Part model, mm, in its own coordinate system. A direction names the side the tool comes from. Give positions to 0.01 mm unless a question says otherwise; leave off trailing zeros. Write each loop counter-clockwise with the first axis right and the second up, starting at its lowest first coordinate (ties: lowest second). Pieces come first, ordered by that corner, then holes.
```python
from build123d import *

# Parameters (mm, degrees)
F0_W      = 38.862
F0_H      = 38.862
F1_DEPTH  = 10.668
F2_SIZE   = 7.62
F4_DEPTH  = 6.35
F5_SIZE   = 5.08
F7_DEPTH  = 6.35
F8_R      = 10.9982
F9_DEPTH  = 2.794
F10_R     = 2.5
F11_DEPTH = 20.32
F12_W     = 13.1343230445
F12_H     = 2.3335092461
F13_DEPTH = 10.16
F14_R     = 1.5
F14_R_2   = 1.2067449727
F14_R_3   = 1.3291263225
F14_R_4   = 1.3491824754
F15_DEPTH = 6.35


# Not quite as in the source:
# - a feature names something its author has since deleted; it is built from what else it names


with BuildPart() as f1:
    # F0 (on Top) → F1 (new body, symmetric)
    with BuildSketch(Plane.XY):
        Rectangle(F0_W, F0_H)
    extrude(amount=F1_DEPTH, both=True)

    # F2
    f2_edges = [f1.edges().sort_by_distance(p)[0] for p in [
        (19.431, 19.431, 0),
        (-19.431, 19.431, 0),
        (-19.431, -19.431, 0),
        (19.431, -19.431, 0),
    ]]
    chamfer(f2_edges, length=F2_SIZE)

    # F3 (on face) → F4 (join)
    with BuildSketch(Plane.XY.offset(10.668)):
        Polygon((11.811, 19.431), (-11.811, 19.431), (-19.431, 11.811), (-19.431, -11.811), (-11.811, -19.431), (11.811, -19.431), (19.431, -11.811), (19.431, 11.811), align=None)
        Polygon((19.431, 19.431), (11.811, 19.431), (19.431, 11.811), align=None)
        Polygon((-11.811, 19.431), (-19.431, 19.431), (-19.431, 11.811), align=None)
        Polygon((-11.811, -19.431), (-19.431, -11.811), (-19.431, -19.431), align=None)
        Polygon((19.431, -19.431), (19.431, -11.811), (11.811, -19.431), align=None)
    extrude(amount=F4_DEPTH)

    # F5
    f5_edges = [f1.edges().sort_by_distance(p)[0] for p in [
        (19.431, 19.431, 13.843),
        (-19.431, 19.431, 13.843),
        (-19.431, -19.431, 13.843),
        (19.431, -19.431, 13.843),
    ]]
    chamfer(f5_edges, length=F5_SIZE)

    # F6 (on face) → F7 (join)
    with BuildSketch(Plane(origin=(0, 0, -10.668), x_dir=(1, 0, 0), z_dir=(0, 0, -1))):
        Polygon((-11.811, 19.431), (-14.351, 19.431), (-19.431, 14.351), (-19.431, 11.811), align=None)
        Polygon((14.351, 19.431), (11.811, 19.431), (19.431, 11.811), (19.431, 14.351), align=None)
        Polygon((19.431, -14.351), (19.431, -11.811), (11.811, -19.431), (14.351, -19.431), align=None)
        Polygon((-11.811, -19.431), (-19.431, -11.811), (-19.431, -14.351), (-14.351, -19.431), align=None)
        Polygon((11.811, 19.431), (-11.811, 19.431), (-19.431, 11.811), (-19.431, -11.811), (-11.811, -19.431), (11.811, -19.431), (19.431, -11.811), (19.431, 11.811), align=None)
    extrude(amount=F7_DEPTH)

    # F8 (on face) + F6 (on face) → F9 (join)
    with BuildSketch(Plane.XY.offset(17.018)):
        Circle(F8_R)
    with BuildSketch(Plane(origin=(0, 0, -10.668), x_dir=(1, 0, 0), z_dir=(0, 0, -1))):
        Polygon((14.351, 19.431), (-14.351, 19.431), (-19.431, 14.351), (-19.431, -14.351), (-14.351, -19.431), (14.351, -19.431), (19.431, -14.351), (19.431, 14.351), align=None)
    extrude(amount=F9_DEPTH, dir=(0, 0, 1))

    # F10 (on face) → F11 (join)
    with BuildSketch(Plane.XY.offset(19.812)):
        Circle(F10_R)
    extrude(amount=F11_DEPTH)

    # F12 (on face) → F13 (cut)
    with BuildSketch(Plane.XY.offset(40.132)):
        with Locations((-0.0065014465, 6.166754623)):
            Rectangle(F12_W, F12_H)
    extrude(amount=-F13_DEPTH, mode=Mode.SUBTRACT)

    # F14 (on face) → F15 (cut)
    with BuildSketch(Plane.XY.offset(17.018)):
        with Locations((-15.5, 15.494)):
            Circle(F14_R)
        with Locations((15.494, 15.494)):
            Circle(F14_R_2)
        with Locations((15.494, -15.494)):
            Circle(F14_R_3)
        with Locations((-15.494, -15.494)):
            Circle(F14_R_4)
    extrude(amount=-F15_DEPTH, mode=Mode.SUBTRACT)


solid = f1.part
```
1) Saw through at A-A, the plane z = -2.5. Write the cut outline in (x, y), then the cut area to 3 significant figures.
Answers follow:
outline: (-19.43, -11.81) - (-11.81, -19.43) - (11.81, -19.43) - (19.43, -11.81) - (19.43, 11.81) - (11.81, 19.43) - (-11.81, 19.43) - (-19.43, 11.81) - close
area: 1,390 mm2
2) Saw through at B-B, the plane x = -15.5. Write the cut outline in (y, z).
Answers follow:
outline: (-18.28, -17.02) - (18.28, -17.02) - (18.28, -7.87) - (15.74, -7.87) - (15.74, 10.67) - (13.99, 10.67) - (13.99, 17.02) - (-14.14, 17.02) - (-14.14, 10.67) - (-15.74, 10.67) - (-15.74, -7.87) - (-18.28, -7.87) - close; (-18.28, 10.67) - (-16.84, 10.67) - (-16.84, 17.02) - (-18.28, 17.02) - close; (16.99, 10.67) - (18.28, 10.67) - (18.28, 17.02) - (16.99, 17.02) - close
3) Pin check, flat tips, straight feed: pin 1 Ø8.5 at (x, y) = (-15, 17.5) entering from +Z; pin 2 Ø0.8 at (x, y) = (-15, 15) entering from +Z. Stop position of each tip, or through.
Answers follow:
pin 1: stops at z = 17.02
pin 2: stops at z = 10.67
4) Wall check: L1, parallel to Y at x = 16.5, z = 11; L2, parallel to Z at x = 13, y = 18.5; L3, parallel to Z at x = 4, y = -15.5. Give the ranges that are in metal, low to high.
Answers follow:
L1: y = -17.28 to -16.36, -14.63 to 14.83, 16.16 to 17.28
L2: z = -17.02 to -7.87, 10.67 to 17.02
L3: z = -17.02 to 17.02
5) 3-axis set-ups, long thin cutter, end or side, ignore diameter. For faces 4 (the face through (-9, 9, 17.018)), 5 (the face through (16, 16, -7.874)), 6 (the face through (16, -17, 10.668)), 7 (the face through (-16, 16, -7.874)), 8 (the face through (-15.57, -15.67, 1.27)): which of +Z, -Z, +X, -X, +Y, -Y reach the whole face in a straight line?
Answers follow:
face 4: +Z
face 5: +X, +Y
face 6: +X, -Y
face 7: -X, +Y
face 8: -X, -Y
6) Two-plate mould, pull along Y, no slides. Class faces 1 (the face through (19.431, 0, 0)), 2 (the face through (-8.73, -6.69, 18.4)), 3 (the face through (-15, -15, 10.668)): +Y half, -Y half, draft (parallel to the pull), parting line (faces both ways), or undercut.
Answers follow:
face 1: draft
face 2: parting line
face 3: undercut
7) Saw through at C-C, the plane y = 0. Write the cut outline in (x, z).
Answers follow:
outline: (-19.43, -17.02) - (19.43, -17.02) - (19.43, 17.02) - (11, 17.02) - (11, 19.81) - (2.5, 19.81) - (2.5, 40.13) - (-2.5, 40.13) - (-2.5, 19.81) - (-11, 19.81) - (-11, 17.02) - (-19.43, 17.02) - close
